Read the model definition and answer for the solid it produces. Units are mm, in the model's axes. Face numbers are marked on the shaded views. Coordinates: 2 decimals unless noted, no trailing zeros. Loops run counter-clockwise (first coordinate to the right, second up) from the corner with the lowest first, then second, coordinate; pieces in that order, holes last.
from build123d import *

# Parameters (mm, degrees)
F0_R     = 12.7
F1_DEPTH = 90.17
F2_R     = 7.62
F3_T     = -2.54


# Not quite as in the source:
# - a shell that OpenCascade refuses in one call is made with other operations: the cavity is built on its own and cut out


with BuildPart() as f1:
    # F0 (on Front) → F1 (new body)
    with BuildSketch(Plane.XZ):
        Circle(F0_R)
    extrude(amount=F1_DEPTH)

    # F2
    f2_edges = [f1.edges().sort_by_distance(p)[0] for p in [
        (-12.7, -90.17, 0),
        (-12.7, 0, 0),
    ]]
    fillet(f2_edges, radius=F2_R)

    # F3: a shell. OpenCascade refuses it in one call, so the cavity is built on its own and cut out:
    # the body offset inwards by the wall thickness, plus a prism from it out through each open face.
    f3_core = offset(f1.part, amount=F3_T, mode=Mode.PRIVATE)
    f3_exits = [f3_core.faces().sort_by_distance(p)[0] for p in [
        (0, -87.63, 0),
    ]]
    add(f3_core, mode=Mode.SUBTRACT)
    extrude(f3_exits, amount=-F3_T, mode=Mode.SUBTRACT)


solid = f1.part
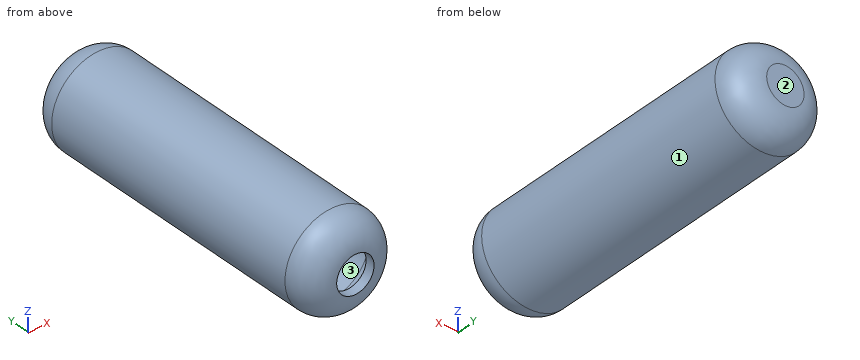
Q1. A cutting plane is placed at A-A (y = -28.5). Give the vertices of the cut face in (x, z), then the cut area to 3 significant figures.
Findings below:
outline: circle Ø25.4 at (0, 0); hole circle Ø20.32 at (0, 0)
area: 182 mm2
Q2. Straight lines are drawn through the part: probe 1 along Z at (x, y) = (0, -47); probe 2 along Y at (x, z) = (-2.75, -3); probe 3 along X at (y, z) = (-11, 7.5). For each, find the intervals that lie inside material, in ascending order.
Findings below:
probe 1: z = -12.7 to -10.16, 10.16 to 12.7
probe 2: y = -2.54 to 0
probe 3: x = -10.25 to -6.85, 6.85 to 10.25
Q3. Determine the mould class of the marked faces 1, 2 and 3 for opening direction Y: +Y half, -Y half, draft (parallel to the pull), parting line (faces both ways), or undercut.
Findings below:
face 1: draft
face 2: +Y half
face 3: undercut
Q4. Flat-ended cylindrical pins translate along their axes: pin 1 Ø1.5 at (x, z) = (-7, -9) entering from -Y; pin 2 Ø4 at (x, z) = (1, -4) entering from -Y; pin 3 Ø5 at (x, y) = (-3, -69.5) entering from +Z; pin 4 Ø1 at (x, y) = (-9, -17.5) entering from +Z. Find the tip coordinate at first contact, or state that the pin passes through.
Findings below:
pin 1: stops at y = -87.75
pin 2: stops at y = -90.17
pin 3: stops at z = 12.69
pin 4: stops at z = 9.44
